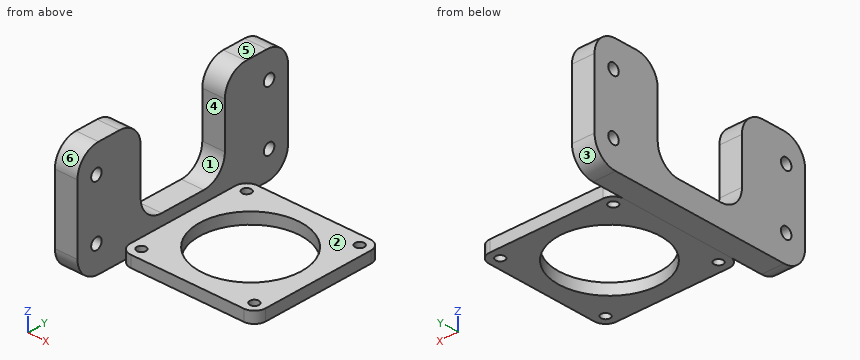
```python
from build123d import *

# Parameters (mm, degrees)
SKETCH2_R           = 2
SKETCH2_R_2         = 22.5
BOSS_EXTRUDE2_DEPTH = 5
SKETCH3_R           = 2.5
BOSS_EXTRUDE3_DEPTH = 10


with BuildPart() as part:
    # Sketch2 → Boss-Extrude2 (new body)
    with BuildSketch(Plane.XY):
        with BuildLine():
            Line((25, 30), (-25, 30))
            ThreePointArc((-25, 30), (-28.535533906, 28.535533906), (-30, 25))
            Line((-30, 25), (-30, -25))
            ThreePointArc((-30, -25), (-28.535533906, -28.535533906), (-25, -30))
            Line((-25, -30), (25, -30))
            ThreePointArc((25, -30), (28.535533906, -28.535533906), (30, -25))
            Line((30, -25), (30, 25))
            ThreePointArc((30, 25), (28.535533906, 28.535533906), (25, 30))
        make_face()
        with Locations((-25, 25)):
            Circle(SKETCH2_R, mode=Mode.SUBTRACT)
        with Locations((25, 25)):
            Circle(SKETCH2_R, mode=Mode.SUBTRACT)
        with Locations((25, -25)):
            Circle(SKETCH2_R, mode=Mode.SUBTRACT)
        with Locations((-25, -25)):
            Circle(SKETCH2_R, mode=Mode.SUBTRACT)
        Circle(SKETCH2_R_2, mode=Mode.SUBTRACT)
    extrude(amount=BOSS_EXTRUDE2_DEPTH)

    # Sketch3 → Boss-Extrude3 (add)
    with BuildSketch(Plane.ZY.offset(30)):
        with BuildLine():
            Line((39.932932244, 50), (9.932932244, 50))
            ThreePointArc((9.932932244, 50), (2.861864432, 47.071067812), (-0.067067756, 40))
            Line((-0.067067756, 40), (-0.067067756, -40))
            ThreePointArc((-0.067067756, -40), (2.861864432, -47.071067812), (9.932932244, -50))
            Line((9.932932244, -50), (39.932932244, -50))
            ThreePointArc((39.932932244, -50), (47.004000055, -47.071067812), (49.932932244, -40))
            Line((49.932932244, -40), (49.932932244, -30))
            ThreePointArc((49.932932244, -30), (47.004000055, -22.928932188), (39.932932244, -20))
            Line((39.932932244, -20), (19.932932244, -20))
            ThreePointArc((19.932932244, -20), (12.861864432, -17.071067812), (9.932932244, -10))
            Line((9.932932244, -10), (9.932932244, 10))
            ThreePointArc((9.932932244, 10), (12.861864432, 17.071067812), (19.932932244, 20))
            Line((19.932932244, 20), (39.932932244, 20))
            ThreePointArc((39.932932244, 20), (47.004000055, 22.928932188), (49.932932244, 30))
            Line((49.932932244, 30), (49.932932244, 40))
            ThreePointArc((49.932932244, 40), (47.004000055, 47.071067812), (39.932932244, 50))
        make_face()
        with Locations((11.932932244, -41)):
            Circle(SKETCH3_R, mode=Mode.SUBTRACT)
        with Locations((37.932932244, -41)):
            Circle(SKETCH3_R, mode=Mode.SUBTRACT)
        with Locations((11.932932244, 41)):
            Circle(SKETCH3_R, mode=Mode.SUBTRACT)
        with Locations((37.932932244, 41)):
            Circle(SKETCH3_R, mode=Mode.SUBTRACT)
    extrude(amount=BOSS_EXTRUDE3_DEPTH)


solid = part.part
```
Design review of the part built by this model. Coordinates are the model's own, in mm. Face numbers are marked on the shaded views. A direction names the side the tool comes from. Give positions to 0.01 mm unless a question says otherwise; leave off trailing zeros. Order: outer loops, then holes, each group sorted by start corner. A loop starts at its lowest first (then second) coordinate and runs counter-clockwise, first axis right, second up. Notation, with made-up numbers: M -28.75,73 L 26.25,73 A28 ccw 26.25,107 Z; hole C 7.5,-10 d7. An arc over 180 degrees is marked long. One line per question, with ' | ' between items. Start each with the question number.
Q1. We need section C-C (z = 29). Write out the cut boundary in (x, y).
Q2. We need section D-D (x = -33.5). Write out the cut boundary in (y, z), plus the area to 3 significant figures.
Q3. The part is to be moulded in two halves that separate along Y. For the marked faces 4, 5 and 6, say which applies: +Y half, -Y half, draft (parallel to the pull), parting line (faces both ways), or undercut.
Q4. We need section A-A (y = 0). Write out the cut boundary in (x, z).
Q5. Machinability: for the marked faces 1, 2 and 3, which of the approach directions +Z, -Z, +X, -X, +Y, -Y give a long, thin tool a straight path to every point of the face, cutting with its end or side? Answer none if there is none.
Q6. For pin 1 Ø4.5 at (y, z) = (41, 37.93) entering from -X; pin 2 Ø15 at (y, z) = (-22, 18.5) entering from +X; pin 3 Ø5 at (x, y) = (-10.5, -18) entering from +Z; pin 4 Ø2.5 at (x, z) = (-8.5, 3) entering from +Y, all flat-tipped, find the tip position at first contact; note any pin that passes through.
Q7. We need section B-B (x = 0). Write out the cut boundary in (y, z), plus the area to 3 significant figures.
Q8. For L1, parallel to Y at x = 25, z = 3; L2, parallel to X at y = 38, z = 8; L3, parallel to Z at x = -16.5, y = 19.5, list the stretches that pass through material, from the lowest coordinate up. Write a range as [from, to].
Returned:
1) outline: M -40,-50 L -30,-50 L -30,-20 L -40,-20 Z; M -40,20 L -30,20 L -30,50 L -40,50 Z
2) outline: M -50,9.93 A10 ccw -40,-0.07 L 40,-0.07 A10 ccw 50,9.93 L 50,39.93 A10 ccw 40,49.93 L 30,49.93 A10 ccw 20,39.93 L 20,19.93 A10 cw 10,9.93 L -10,9.93 A10 cw -20,19.93 L -20,39.93 A10 ccw -30,49.93 L -40,49.93 A10 ccw -50,39.93 Z; hole C -41,11.93 d5; hole C -41,37.93 d5; hole C 41,11.93 d5; hole C 41,37.93 d5 | area: 3,240 mm2
3) face 4: undercut | face 5: draft | face 6: -Y half
4) outline: M -40,-0.07 L -30,-0.07 L -30,0 L -22.5,0 L -22.5,5 L -30,5 L -30,9.93 L -40,9.93 Z; M 22.5,0 L 30,0 L 30,5 L 22.5,5 Z
5) face 1: +Z, +X, -X | face 2: +Z, +X, +Y, -Y | face 3: -Z, +X, -X, +Y
6) pin 1: through | pin 2: x = -30 | pin 3: z = 5 | pin 4: y = 30
7) outline: M -30,0 L -22.5,0 L -22.5,5 L -30,5 Z; M 22.5,0 L 30,0 L 30,5 L 22.5,5 Z | area: 75.0 mm2
8) L1: [-30, -27], [-23, 23], [27, 30] | L2: [-40, -30] | L3: [0, 5]
